Part model, mm, in its own coordinate system. A direction names the side the tool comes from. Round coordinates to 2 decimals unless told otherwise and drop trailing zeros. Write each loop counter-clockwise with the first axis right and the second up, starting at its lowest first coordinate (ties: lowest second). Pieces come first, ordered by that corner, then holes. Notation, with made-up numbers: M -13,33 L 22,33 A34 cw 22,65 Z; hole C 55.25,32 d7. An arc over 180 degrees is marked long. Answer as a JSON object with one key per item and string values. Group by question number.
1. Drill centre lines: line 1 (Y direction, x = -1, z = -68); line 2 (Z direction, x = 6, y = 16); line 3 (X direction, y = -0.5, z = -13.5). Where is each one in solid material? Low to high. Write a range as from..to.
2. Band-saw the part on A-A, the plane y = 0. Count the separate pieces of the cut face and the enclosed holes in it, plus the area to 3 significant figures.
3. Two-plate mould, pull along Z, no slides. Class faces 6 (the face through (0, -5, 0)), 7 (the face through (13.081, 0, -72)), 8 (the face through (-12.89, 0.04, -74.23)): +Z half, -Z half, draft (parallel to the pull), parting line (faces both ways), or undercut.
4. Which spindle directions (+Z, -Z, +X, -X, +Y, -Y) get a long thin tool onto all of the face, cutting with end or side? Do faces 1 (the face through (12.89, 0.04, -74.23)), 2 (the face through (-0.33, -2.52, 3.76)), 3 (the face through (0, 0, 7.62)), 4 (the face through (12.7, 0, -72)), 5 (the face through (-13.081, 0, -72)). Say none if no direction does.
5. Band-saw the part on D-D, the plane y = 18. Write the cut outline in (x, z), plus the area to 3 significant figures.
6. Band-saw the part on B-B, the plane x = 0. Write the cut outline in (y, z) (3 decimals).
7. Band-saw the part on C-C, the plane z = -58.5. Write the cut outline in (x, y) (3 decimals), plus the area to 3 significant figures.
8. Drop flat-ended pins along their axis: pin 1 (4 mm diameter, centred on x = 1, y = 1.5, fed in from -Z); pin 2 (8 mm diameter, centred on x = -18.5, z = -64, fed in from +Y); pin 3 (6 mm diameter, centred on y = 3.5, z = -64.5, fed in from -X). Give the stop position or say it passes through.
Autodesk Inventor part; units mm, degrees
ref_plane "YZ Plane" through (0, 0, 0) normal (1, 0, 0) x (0, 1, 0)
ref_plane "XZ Plane" through (0, 0, 0) normal (0, 1, 0) x (-1, 0, 0)
ref_plane "XY Plane" through (0, 0, 0) normal (0, 0, 1) x (1, 0, 0)
sketch "Sketch1" plane through (0, 0, 0) normal (0, 0, 1) x (1, 0, 0)
  circle A0 centre (0, 0) radius 23.495
  dimension "d0" = 46.99
extrude "Extrusion1" add sketch "Sketch1" against normal blind 71.374
sketch "Sketch2" plane through (0, 0, 0) normal (0, 0, 1) x (1, 0, 0)
  circle A0 centre (0, 0) radius 23.495
  circle A1 centre (0, 0) radius 2.54
  dimension "d3" = 5.08
extrude "Extrusion2" add sketch "Sketch2" along normal blind 7.62 contours A1
sketch "Sketch3" plane through (0, 0, -71.374) normal (0, 0, -1) x (-1, 0, 0)
  circle A0 centre (0, 0) radius 23.495
  line L0 (-13.081, 1.651) -> (-12.7, 1.651)
  line L1 (-12.7, 1.651) -> (-12.7, -1.651)
  line L2 (-12.7, -1.651) -> (-13.081, -1.651)
  line L3 (-13.081, -1.651) -> (-13.081, 1.651)
  line L4 (12.7, 1.651) -> (13.081, 1.651)
  line L5 (13.081, 1.651) -> (13.081, -1.651)
  line L6 (13.081, -1.651) -> (12.7, -1.651)
  line L7 (12.7, -1.651) -> (12.7, 1.651)
  dimension "d6" = 3.302
  dimension "d7" = 3.302
  dimension "d8" = 0.381
  dimension "d9" = 0.381
  dimension "d10" = 1.651
  dimension "d11" = 0
  dimension "d12" = 25.4
  dimension "d13" = 12.7
extrude "Extrusion3" add sketch "Sketch3" along normal blind 3.81 contours L0 L1 L2 L3 | L4 L5 L6 L7
sketch "Sketch4" plane through (-13.081, -1.651, -71.374) normal (-1, 0, 0) x (0, 0, 1)
  line L0 (0, 3.302) -> (-3.81, 3.302)
  circle A0 centre (-1.905, 1.651) radius 0.9525
  point P0 (71.374, 1.651)
  dimension "d16" = 1.905
  dimension "d17" = 0.6985
extrude "Extrusion4" cut sketch "Sketch4" against normal blind 127
properties part number "RS775 18v"
Worked answers:
{
 "1": {"line 1": "y = -23.47..23.47", "line 2": "z = -71.37..0", "line 3": "x = -23.49..23.49"},
 "2": {"separate pieces": "3", "enclosed holes": "0", "area": "3,390 mm^2"},
 "3": {"face 6": "+Z half", "face 7": "draft", "face 8": "undercut"},
 "4": {"face 1": "+X, -X", "face 2": "+Z", "face 3": "+Z, +X, -X, +Y, -Y", "face 4": "-Z, +Y, -Y", "face 5": "-Z, -X, +Y, -Y"},
 "5": {"outline": "M -15.1,-71.37 L 15.1,-71.37 L 15.1,0 L -15.1,0 Z", "area": "2,160 mm^2"},
 "6": {"outline": "M -23.495,-71.374 L 23.495,-71.374 L 23.495,0 L 2.54,0 L 2.54,7.62 L -2.54,7.62 L -2.54,0 L -23.495,0 Z"},
 "7": {"outline": "C 0,0 d46.99", "area": "1,730 mm^2"},
 "8": {"pin 1": "stops at z = -71.37", "pin 2": "stops at y = 18.49", "pin 3": "stops at x = -23.49"}
}
